Geometry: final body of the model. Coordinates: model frame, mm. A direction names the side the tool comes from. Give positions to 0.01 mm unless a question says otherwise; leave off trailing zeros. Order: outer loops, then holes, each group sorted by start corner. A loop starts at its lowest first (then second) coordinate and runs counter-clockwise, first axis right, second up. Notation, with made-up numbers: (67, 35) -> (111, 35) arc R33 ccw to (111, 66) -> close; hole circle Ø5 at (-12.5, 65). An arc over 180 degrees is marked (long way). One line per question, with ' | ' between items. Start each with the question number.
(1) First-contact query: pin 1 Ø6 at (x, y) = (-13.5, -57) entering from -Z; pin 2 Ø2 at (x, y) = (12.5, 50) entering from +Z. Flat tips, straight axial feed; report the tip coordinate or a pass-through.
(2) Mould query, pull axis X, two halves, no side actions, for faces 3 (the face through (-0.2, -75, 2.7)), 4 (the face through (-50, -1, 15)), 5 (the face through (-47, -1, 16)), 6 (the face through (50, -1, 15)). Classes: +X half, -X half, draft (parallel to the pull), parting line (faces both ways), or undercut.
(3) Set-up query: faces 1 (the face through (47, -1, 16)), 2 (the face through (12.175, -36.464, 1.521)). Return all of +Z, -Z, +X, -X, +Y, -Y with unobstructed straight access to the full face (end or side cutting, diameter ignored); none if empty.
(4) Ray query, L1, parallel to Y at x = 12.5, z = 1.45; L2, parallel to X at y = 49, z = 6; L3, parallel to Z at x = 45.5, y = 15. Return the intervals inside material, ascending.
(5) Section A-A (y = -60). Return loops of the section in (x, z), then the cut area to 3 significant figures.
(6) Section D-D (y = 51.5). Return loops of the section in (x, z), then the cut area to 3 significant figures.
(7) Section B-B (z = 17.5). Return loops of the section in (x, y).
(8) Section C-C (x = -12.5). Return loops of the section in (y, z), then the cut area to 3 significant figures.
```python
from build123d import *

# Parameters (mm, degrees)
SKETCH1_W           = 100
SKETCH1_H           = 150
BOSS_EXTRUDE1_DEPTH = 30
SHELL1_T            = -3
CUT_EXTRUDE2_REACH  = 96.096
SKETCH2_R           = 1.5


with BuildPart() as part:
    # Sketch1 → Boss-Extrude1 (new body)
    with BuildSketch(Plane.XY):
        Rectangle(SKETCH1_W, SKETCH1_H)
    extrude(amount=BOSS_EXTRUDE1_DEPTH)

    # Shell1
    shell1_openings = [part.faces().sort_by_distance(p)[0] for p in [
        (0, 0, 30),
        (0, 75, 15),
        (0, -75, 15),
    ]]
    offset(amount=SHELL1_T, openings=shell1_openings, kind=Kind.INTERSECTION)

    # Sketch2 → Cut-Extrude2 (cut, up to next)
    with BuildSketch(Plane.XY.offset(3), mode=Mode.PRIVATE) as cut_extrude2_sk1:
        with Locations((-12.5, -35)):
            Circle(SKETCH2_R)
    cut_extrude2_tool1 = extrude(cut_extrude2_sk1.sketch, amount=-CUT_EXTRUDE2_REACH, mode=Mode.PRIVATE) & part.part
    # Sketch2 → Cut-Extrude2 (cut, up to next)
    with BuildSketch(Plane.XY.offset(3), mode=Mode.PRIVATE) as cut_extrude2_sk2:
        with Locations((-12.5, -60)):
            Circle(SKETCH2_R)
    cut_extrude2_tool2 = extrude(cut_extrude2_sk2.sketch, amount=-CUT_EXTRUDE2_REACH, mode=Mode.PRIVATE) & part.part
    # Sketch2 → Cut-Extrude2 (cut, up to next)
    with BuildSketch(Plane.XY.offset(3), mode=Mode.PRIVATE) as cut_extrude2_sk3:
        with Locations((12.5, -60)):
            Circle(SKETCH2_R)
    cut_extrude2_tool3 = extrude(cut_extrude2_sk3.sketch, amount=-CUT_EXTRUDE2_REACH, mode=Mode.PRIVATE) & part.part
    # Sketch2 → Cut-Extrude2 (cut, up to next)
    with BuildSketch(Plane.XY.offset(3), mode=Mode.PRIVATE) as cut_extrude2_sk4:
        with Locations((12.5, -35)):
            Circle(SKETCH2_R)
    cut_extrude2_tool4 = extrude(cut_extrude2_sk4.sketch, amount=-CUT_EXTRUDE2_REACH, mode=Mode.PRIVATE) & part.part
    add(cut_extrude2_tool1.solids().sort_by_distance((-12.5, -35, 3))[0], mode=Mode.SUBTRACT)
    add(cut_extrude2_tool2.solids().sort_by_distance((-12.5, -60, 3))[0], mode=Mode.SUBTRACT)
    add(cut_extrude2_tool3.solids().sort_by_distance((12.5, -60, 3))[0], mode=Mode.SUBTRACT)
    add(cut_extrude2_tool4.solids().sort_by_distance((12.5, -35, 3))[0], mode=Mode.SUBTRACT)


solid = part.part
```
Response:
1) pin 1: stops at z = 0 | pin 2: stops at z = 3
2) face 3: draft | face 4: -X half | face 5: undercut | face 6: +X half
3) face 1: +Z, +Y, -Y | face 2: +Z, -Z
4) L1: y = -75 to -61.5, -58.5 to -36.5, -33.5 to 75 | L2: x = -50 to -47, 47 to 50 | L3: z = 0 to 3
5) outline: (-50, 0) -> (-14, 0) -> (-14, 3) -> (-47, 3) -> (-47, 30) -> (-50, 30) -> close; (-11, 0) -> (11, 0) -> (11, 3) -> (-11, 3) -> close; (14, 0) -> (50, 0) -> (50, 30) -> (47, 30) -> (47, 3) -> (14, 3) -> close | area: 444 mm^2
6) outline: (-50, 0) -> (50, 0) -> (50, 30) -> (47, 30) -> (47, 3) -> (-47, 3) -> (-47, 30) -> (-50, 30) -> close | area: 462 mm^2
7) outline: (-50, -75) -> (-47, -75) -> (-47, 75) -> (-50, 75) -> close; (47, -75) -> (50, -75) -> (50, 75) -> (47, 75) -> close
8) outline: (-75, 0) -> (-61.5, 0) -> (-61.5, 3) -> (-75, 3) -> close; (-58.5, 0) -> (-36.5, 0) -> (-36.5, 3) -> (-58.5, 3) -> close; (-33.5, 0) -> (75, 0) -> (75, 3) -> (-33.5, 3) -> close | area: 432 mm^2
